```python
from build123d import *


with BuildPart() as part:
    # Sketch1 → Revolve1 (revolve)
    with BuildSketch(Plane.XY, mode=Mode.PRIVATE) as revolve1_sk:
        with BuildLine():
            ThreePointArc((8.25, -32), (8.103553391, -32.353553391), (7.75, -32.5))
            Line((7.75, -32.5), (7.25, -32.5))
            ThreePointArc((7.25, -32.5), (3.834465413, -34.357449696), (0, -35))
            Line((0, -35), (0, 0))
            Line((0, 0), (2, 0))
            ThreePointArc((2, 0), (2.353553391, -0.146446609), (2.5, -0.5))
            Line((2.5, -0.5), (2.5, -17.5))
            ThreePointArc((2.5, -17.5), (2.646446609, -17.853553391), (3, -18))
            Line((3, -18), (6.042893219, -18))
            ThreePointArc((6.042893219, -18), (6.234234935, -18.038060234), (6.396446609, -18.146446609))
            Line((6.396446609, -18.146446609), (8.103553391, -19.853553391))
            ThreePointArc((8.103553391, -19.853553391), (8.211939766, -20.015765065), (8.25, -20.207106781))
            Line((8.25, -20.207106781), (8.25, -32))
        make_face()
    revolve(revolve1_sk.sketch.rotate(Axis((0, 0, 0), (0, -1, 0)), 180), axis=Axis((0, 0, 0), (0, -1, 0)))


solid = part.part
```
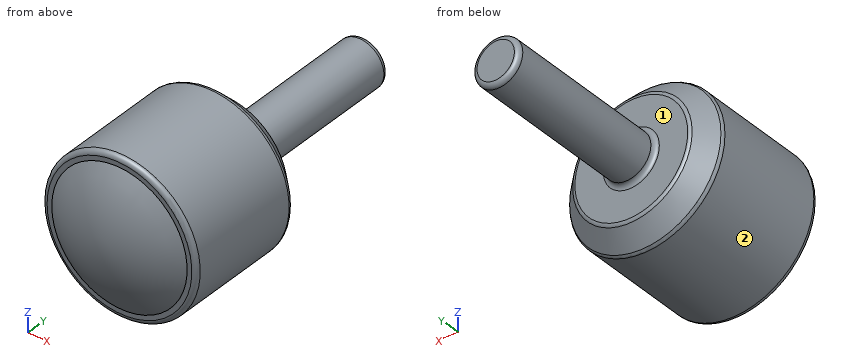
The listing builds one solid part. Answer for the finished solid, in the listing's coordinates (mm). Face numbers are marked on the shaded views. A direction names the side the tool comes from. Give positions to 0.01 mm unless a question says otherwise; leave off trailing zeros. Write each loop counter-clockwise with the first axis right and the second up, starting at its lowest first coordinate (ties: lowest second). Pieces come first, ordered by that corner, then holes. Notation, with made-up numbers: (49.5, -21.75) -> (77.5, -21.75) arc R33 ccw to (77.5, 16.25) -> close; hole circle Ø11 at (-36, 68.5). An arc over 180 degrees is marked (long way). Use one line per item in the form item = value.
1) Section C-C on y = -28 is taken. Write down the section's boundary in (x, z), plus the area to 3 significant figures.
Result:
outline = circle Ø16.5 at (0, 0)
area = 214 mm²
2) A tool of negligible diameter and unlimited length cuts with its end or side. For the marked faces 1 and 2, from which of +Z, -Z, +X, -X, +Y, -Y can it reach the whole face along a straight path? Write none if from no direction.
Result:
face_1 = +Y
face_2 = +Y, -Y
3) Straight lines are drawn through the part: probe 1 along X at (y, z) = (-25, 0.25); probe 2 along Y at (x, z) = (3.75, -5.25); probe 3 along X at (y, z) = (-33, 2.75). For each, find the intervals that lie inside material, in ascending order.
Result:
probe_1 = -8.25 to 8.25
probe_2 = -33.07 to -18.2
probe_3 = -5.96 to 5.96
4) Each of these flat-tipped pins is pushed along its axis until it touches: P1, Ø8, axis at y = -18.5, z = -5, coming from the -X side; P2, Ø6, axis at x = -3.5, z = -6.5, coming from the -Y side; P3, Ø3, axis at x = -3.5, y = -25, coming from the +Z side. Where does it stop, or does it pass through?
Result:
P1 = -8.13
P2 = -34.15
P3 = 8
